```python
from build123d import *

# Parameters (mm, degrees)
BASPROSKE_W        = 10
BASPROSKE_H        = 22
TOOTHCUT_DEPTH     = 33.680269277
TEETHCUTS_COUNT    = 20
TEETHCUTS_ANGLE    = 342
BORSKE_R           = 0.4
BORE_DEPTH         = 50.0000508
CUT_EXTRUDE1_DEPTH = 6
SKETCH2_R          = 2
CUT_EXTRUDE2_DEPTH = 6
CUT_EXTRUDE3_DEPTH = 6


with BuildPart() as part:
    # BasProSke → Base-Revolve (revolve)
    with BuildSketch(Plane(origin=(0, 0, 0), x_dir=(1, 0, 0), z_dir=(0, 1, 0)), mode=Mode.PRIVATE) as base_revolve_sk:
        with Locations((5, 11)):
            Rectangle(BASPROSKE_W, BASPROSKE_H)
    revolve(base_revolve_sk.sketch.rotate(Axis((-10, 0, 0), (1, 0, 0)), 180), axis=Axis((-10, 0, 0), (1, 0, 0)))

    # TooCutSke → ToothCut (cut, through all)
    with BuildSketch(Plane(origin=(0, 0, 0), x_dir=(0, 0, -1), z_dir=(1, 0, 0))):
        with BuildLine():
            ThreePointArc((0.986171591, 17.471189616), (0, 17.499), (-0.986171591, 17.471189616))
            ThreePointArc((-0.986171591, 17.471189616), (-1.626916196, 19.798789858), (-2.932850173, 21.829260982))
            ThreePointArc((-2.932850173, 21.829260982), (0, 22.0254), (2.932850173, 21.829260982))
            ThreePointArc((2.932850173, 21.829260982), (1.626916196, 19.798789858), (0.986171591, 17.471189616))
        make_face()
    toothcut = extrude(amount=TOOTHCUT_DEPTH, mode=Mode.SUBTRACT)

    # TeethCuts: ToothCut ×20 about axis
    teethcuts_axis = Axis((-10, 0, 0), (1, 0, 0))
    for i in range(1, TEETHCUTS_COUNT):
        add(toothcut.rotate(teethcuts_axis, i * TEETHCUTS_ANGLE / (TEETHCUTS_COUNT - 1)), mode=Mode.SUBTRACT)

    # BorSke → Bore (cut, symmetric)
    with BuildSketch(Plane(origin=(0, 0, 0), x_dir=(0, 0, -1), z_dir=(1, 0, 0))):
        with Locations(Location((0, 0, 0), (0, 0, 180))):
            Circle(BORSKE_R)
    extrude(amount=BORE_DEPTH, both=True, mode=Mode.SUBTRACT)

    # Sketch1 → Cut-Extrude1 (cut)
    with BuildSketch(Plane.ZY):
        Polygon((-5.947236483, -3.553917279), (0.104168329, -6.927416915), (6.05140712, -3.373496436), (5.947241098, 3.553923678), (-0.104163715, 6.927423314), (-6.051402506, 3.373502835), align=None)
    extrude(amount=-CUT_EXTRUDE1_DEPTH, mode=Mode.SUBTRACT)

    # Sketch2 → Cut-Extrude2 (cut)
    with BuildSketch(Plane(origin=(10, 0, 0), x_dir=(0, 0, -1), z_dir=(1, 0, 0))):
        with Locations((-2.307e-06, 3.199e-06)):
            Circle(SKETCH2_R)
    extrude(amount=-CUT_EXTRUDE2_DEPTH, mode=Mode.SUBTRACT)

    # Sketch4 → Cut-Extrude3 (cut)
    with BuildSketch(Plane.ZY):
        Polygon((-6.346541022, 3.518535779), (-6.237773669, -3.714889608), (0.071344514, -7.232057695), (6.334133484, -3.489572357), (6.225545747, 3.731907869), (-0.094007056, 7.254892984), align=None)
    extrude(amount=-CUT_EXTRUDE3_DEPTH, mode=Mode.SUBTRACT)


solid = part.part
```
Input: part model. Units: mm. Frame: model coordinates. A direction names the side the tool comes from. Round coordinates to 2 decimals unless told otherwise and drop trailing zeros. Loops run counter-clockwise (first coordinate to the right, second up) from the corner with the lowest first, then second, coordinate; pieces in that order, holes last. Notation, with made-up numbers: (-37, 40.5) -> (19, 40.5) arc R18 cw to (19, 72.5) -> close; hole circle Ø5 at (59, 88). An arc over 180 degrees is marked (long way). Use one line per item in the form item = value. Start each with the question number.
Item 1: Material intervals for L1, parallel to Z at x = 6.75, y = 18; L2, parallel to Z at x = 8.25, y = 19.5; L3, parallel to Y at x = 9.25, z = 3, sorted ascending. Write a range as from..to.
Item 2: Section query B-B on z = 12. Return the cut outline in (x, y).
Item 3: Set-up query: faces 1 (the face through (4.93, -18.341, 7.678)), 2 (the face through (4.93, -7.63, 18.29)), 3 (the face through (3, 5.4, -3.2)). Return all of +Z, -Z, +X, -X, +Y, -Y with unobstructed straight access to the full face (end or side cutting, diameter ignored); none if empty.
Item 4: Mould query, pull axis Y, two halves, no side actions, for faces 4 (the face through (4.93, 15.037, 12.911)), 5 (the face through (4.93, -7.678, -18.341)), 6 (the face through (5.07, -3.449, -21.728)). Classes: pulls with the +Y half, pulls with the -Y half, needs draft (parallel to the pull), parting line crosses it, or undercut.
Item 5: Section query C-C on z = -13. Return the cut outline in (x, y).
Item 6: Contact query for flat-ended pins moving along their axis: pin 1 Ø6.5 at (y, z) = (-2.5, -1.5) entering from -X; pin 2 Ø5 at (x, y) = (3.5, -17.5) entering from +Z; pin 3 Ø2 at (x, z) = (3, 16.5) entering from +Y; pin 4 Ø2.5 at (y, z) = (0, 0) entering from -X. Output: stop coordinate, or through.
Item 7: Section query A-A on y = 0. Return the cut outline in (x, z), then the cut area to 3 significant figures.
Ans:
q1.L1 = -10.47..-7.39, -4.6..-1.07, 1.07..4.6, 7.39..10.47
q1.L2 = -10.19..-8.99, -4.55..-1.5, 1.5..4.55, 8.99..10.19
q1.L3 = -21.79..21.79
q2.outline = (0, -14.42) -> (10, -14.42) -> (10, 14.42) -> (0, 14.42) -> close
q3.face_1 = +X, -X, -Y
q3.face_2 = +Z, +X, -X
q3.face_3 = -X
q4.face_4 = pulls with the +Y half
q4.face_5 = undercut
q4.face_6 = pulls with the -Y half
q5.outline = (0, -15.09) -> (10, -15.09) -> (10, 15.09) -> (0, 15.09) -> close
q6.pin_1 = 6
q6.pin_2 = 15.93
q6.pin_3 = 15.61
q6.pin_4 = through
q7.outline = (0, -17.5) -> (10, -17.5) -> (10, -2) -> (6, -2) -> (6, -6.29) -> (0, -6.29) -> close; (0, 6.28) -> (6, 6.28) -> (6, 2) -> (10, 2) -> (10, 17.5) -> (0, 17.5) -> close
q7.area = 259 mm^2
